from build123d import *

# Parameters (mm, degrees)
SKETCH1_W           = 10
SKETCH1_H           = 3
SKETCH1_W_2         = 3
SKETCH1_H_2         = 10
BOSS_EXTRUDE1_DEPTH = 3


with BuildPart() as part:
    # Sketch1 → Boss-Extrude1 (new body)
    with BuildSketch(Plane(origin=(0, 0, 0), x_dir=(1, 0, 0), z_dir=(0, 1, 0))):
        Polygon((0, 0), (0, 5), (-3, 5), (-3, 15), (0, 15), (0, 25), (-3, 25), (-3, 35), (0, 35), (0, 40), (4.642383454, 38.143046618), (5.756555483, 40.928476691), (15.041322392, 37.214569927), (13.927150363, 34.429139855), (36.072849637, 25.570860145), (37.187021666, 28.356290218), (46.471788575, 24.642383454), (45.357616546, 21.856953382), (50, 20), (50, 0), align=None)
        with Locations((10, 3.5)):
            Rectangle(SKETCH1_W, SKETCH1_H, mode=Mode.SUBTRACT)
        with Locations((35, 3.5)):
            Rectangle(SKETCH1_W, SKETCH1_H, mode=Mode.SUBTRACT)
        with Locations((46.5, 12)):
            Rectangle(SKETCH1_W_2, SKETCH1_H_2, mode=Mode.SUBTRACT)
    extrude(amount=BOSS_EXTRUDE1_DEPTH)


solid = part.part
Check sheet for the modelled part. Datum: model origin and axes. Units: mm. A direction names the side the tool comes from. Give positions to 0.01 mm unless a question says otherwise; leave off trailing zeros. Write each loop counter-clockwise with the first axis right and the second up, starting at its lowest first coordinate (ties: lowest second). Pieces come first, ordered by that corner, then holes. Notation, with made-up numbers: M 15,6.25 L 34,6.25 A34 ccw 34,40.25 Z; hole C 65.25,-17 d7. An arc over 180 degrees is marked long. Use one line per item in the form item = value.
(1) Section check C-C on y = 1.95. State how many separate pieces and enclosed holes the cut face has, plus the area to 3 significant figures.
Answer block:
separate_pieces = 1
enclosed_holes = 3
area = 1,530 mm2
(2) Section check B-B on x = 33. Record the boundary of the cut face in (y, z).
Answer block:
outline = M 0,-26.8 L 3,-26.8 L 3,-5 L 0,-5 Z; M 0,-2 L 3,-2 L 3,0 L 0,0 Z
(3) Section check A-A on z = -12. Record the boundary of the cut face in (x, y).
Answer block:
outline = M -3,0 L 45,0 L 45,3 L -3,3 Z; M 48,0 L 50,0 L 50,3 L 48,3 Z
(4) Depth check by flat-ended pin: P1, Ø1.5, axis at x = 23, y = 1, coming from the +Z side; P2, Ø1.5, axis at x = -1.5, y = 2, coming from the +Z side; P3, Ø1.5, axis at x = -1.5, y = 1.5, coming from the -Z side. Enter the tip coordinate at first touch or a pass-through.
Answer block:
P1 = 0
P2 = -5
P3 = -35
(5) Draft check along X on faces 4 (the flat face through (25, 1, 0)), 5 (the flat face through (48, 1, -12)), 6 (the flat face through (0, 1, -20)), 7 (the flat face through (41.764, 1.479, -26.525)). Enter one of: pulls with the +X half, pulls with the -X half, needs draft (parallel to the pull), parting line crosses it, or undercut.
Answer block:
face_4 = needs draft
face_5 = undercut
face_6 = pulls with the -X half
face_7 = pulls with the +X half
(6) Section check D-D on x = 23.5. Record the boundary of the cut face in (y, z).
Answer block:
outline = M 0,-30.6 L 3,-30.6 L 3,0 L 0,0 Z
(7) Tool access check on faces 1 (the flat face through (36.62, 1.48, -26.94)), 2 (the flat face through (-2, 1, -35)), 3 (the flat face through (35, 1, -2)). Record the directions out of +Z, -Z, +X, -X, +Y, -Y that give a thin tool (end or side, any length) a straight path to the whole face; none if there is none.
Answer block:
face_1 = -Z, +Y, -Y
face_2 = -Z, -X, +Y, -Y
face_3 = +Y, -Y
(8) Material ranges on line 1 along X through (y, z) = (1.7, -11); line 2 along Z through (x, y) = (39, 2.75); line 3 along Z through (x, y) = (8.5, 1.55), recorded low to high.
Answer block:
line_1 = -3 to 45, 48 to 50
line_2 = -27.63 to -5, -2 to 0
line_3 = -39.83 to -5, -2 to 0
